CAD build for the part. Positions are in the model's coordinates, mm. Coordinates: 2 decimals unless noted, no trailing zeros. Loops run counter-clockwise (first coordinate to the right, second up) from the corner with the lowest first, then second, coordinate; pieces in that order, holes last. Notation, with made-up numbers: (51, 89) -> (83, 89) arc R27 cw to (83, 114) -> close; hole circle Ø7 at (-33, 8.25). An arc over 180 degrees is marked (long way). Write item = value, one per line. Start each with the question number.
(1) Band-saw the part on B-B (x = 67.75). Write the cut outline in (y, z), and give its area (3 significant figures).
(2) Pull direction X, two halves, no side cores. Call faces 1 (the face through (80.174, 1.411, 0.258)), 2 (the face through (82.04, -0.43, 0.25)), 3 (the face through (73, -6, 0)), 4 (the face through (69.34, -0.36, 0.26)): +X half, -X half, draft (parallel to the pull), parting line (faces both ways), or undercut.
(3) Drill centre lines: line 1 (X direction, y = -2.5, z = 0.45); line 2 (Y direction, x = 73, z = 0.1); line 3 (X direction, y = 2, z = 0.45). Where is each one in solid material? Low to high. Write a range as from..to.
(4) Band-saw the part on D-D (y = 22.5). Write the cut outline in (x, z), and give its area (3 significant figures).
(5) Band-saw the part on A-A (y = 0). Write the cut outline in (x, z).
(6) Band-saw the part on C-C (z = 0.2). Write the cut outline in (x, y), and give its area (3 significant figures).
```python
from build123d import *

# Parameters (mm, degrees)
SKETCH4_R           = 82.042
BOSS_EXTRUDE2_DEPTH = 0.508
SKETCH5_R           = 69.342
CUT_EXTRUDE5_DEPTH  = 1.508
SKETCH6_R           = 4.699
CUT_EXTRUDE6_DEPTH  = 1.508
SKETCH8_OUTSIDE_W   = 212.494
SKETCH8_OUTSIDE_H   = 212.494
CUT_EXTRUDE11_DEPTH = 1.508


with BuildPart() as part:
    # Sketch4 → Boss-Extrude2 (new body)
    with BuildSketch(Plane.XY):
        Circle(SKETCH4_R)
    extrude(amount=BOSS_EXTRUDE2_DEPTH)

    # Sketch5 → Cut-Extrude5 (cut, through all)
    with BuildSketch(Plane.XY.offset(0.508)):
        Circle(SKETCH5_R)
    extrude(amount=-CUT_EXTRUDE5_DEPTH, mode=Mode.SUBTRACT)

    # Sketch6 → Cut-Extrude6 (cut, through all)
    with BuildSketch(Plane.XY.offset(0.508)):
        with Locations((75.692, 0)):
            Circle(SKETCH6_R)
    extrude(amount=-CUT_EXTRUDE6_DEPTH, mode=Mode.SUBTRACT)

    # Sketch8 outside → Cut-Extrude11 (cut, through all)
    with BuildSketch(Plane.XY.offset(0.508)):
        Rectangle(SKETCH8_OUTSIDE_W, SKETCH8_OUTSIDE_H)
        with BuildLine():
            Line((64.538916848, -25.358256565), (76.273850543, -30.219025255))
            ThreePointArc((76.273850543, -30.219025255), (82.042, 0), (76.273850543, 30.219025255))
            Line((76.273850543, 30.219025255), (64.538916848, 25.358256565))
            ThreePointArc((64.538916848, 25.358256565), (69.342, 0), (64.538916848, -25.358256565))
        make_face(mode=Mode.SUBTRACT)
    extrude(amount=-CUT_EXTRUDE11_DEPTH, mode=Mode.SUBTRACT)


solid = part.part
```
Findings below:
q1.outline = (-26.69, 0) -> (-14.77, 0) -> (-14.77, 0.51) -> (-26.69, 0.51) -> close; (14.77, 0) -> (26.69, 0) -> (26.69, 0.51) -> (14.77, 0.51) -> close
q1.area = 12.1 mm²
q2.face_1 = undercut
q2.face_2 = +X half
q2.face_3 = draft
q2.face_4 = -X half
q3.line_1 = 69.3..71.71, 79.67..82
q3.line_2 = -28.86..-3.85, 3.85..28.86
q3.line_3 = 69.31..71.44, 79.94..82.02
q4.outline = (65.59, 0) -> (78.9, 0) -> (78.9, 0.51) -> (65.59, 0.51) -> close
q4.area = 6.76 mm²
q5.outline = (69.34, 0) -> (70.99, 0) -> (70.99, 0.51) -> (69.34, 0.51) -> close; (80.39, 0) -> (82.04, 0) -> (82.04, 0.51) -> (80.39, 0.51) -> close
q6.outline = (64.54, -25.36) -> (76.27, -30.22) arc R82.04 ccw to (76.27, 30.22) -> (64.54, 25.36) arc R69.34 cw to start; hole circle Ø9.4 at (75.69, 0)
q6.area = 653 mm²
